Part model, mm, in its own coordinate system. Face numbers are marked on the shaded views. A direction names the side the tool comes from. Coordinates: 2 decimals unless noted, no trailing zeros. Loops run counter-clockwise (first coordinate to the right, second up) from the corner with the lowest first, then second, coordinate; pieces in that order, holes last. Notation, with made-up numbers: (86, 75) - (132, 75) arc R24 ccw to (132, 114) - close; hole circle Ø1 at (15.25, -1). An arc over 180 degrees is marked (long way). Answer as CSV lines item,"result".
from build123d import *

# Parameters (mm, degrees)
SKETCH1_W           = 26
SKETCH1_H           = 41
BOSS_EXTRUDE1_DEPTH = 10
SKETCH2_W           = 26
SKETCH2_H           = 5
BOSS_EXTRUDE2_DEPTH = 25
CUT_EXTRUDE1_REACH  = 73.638
CHAMFER1_SIZE       = 2
SKETCH4_W           = 56
SKETCH4_H           = 8
BOSS_EXTRUDE3_DEPTH = 9
CUT_EXTRUDE2_REACH  = 73.386
SKETCH5_R           = 2.15
SKETCH6_R           = 3.5
CUT_EXTRUDE3_DEPTH  = 5
CHAMFER3_SIZE       = 3
CUT_EXTRUDE5_DEPTH  = 1
CUT_EXTRUDE6_DEPTH  = 4
CUT_EXTRUDE7_REACH  = 73.638
SKETCH12_R          = 1.65
SKETCH14_W          = 12
SKETCH14_H          = 12
CUT_EXTRUDE9_DEPTH  = 7


with BuildPart() as part:
    # Sketch1 → Boss-Extrude1 (new body)
    with BuildSketch(Plane(origin=(0, 0, 0), x_dir=(1, 0, 0), z_dir=(0, 1, 0))):
        with Locations((13, 20.5)):
            Rectangle(SKETCH1_W, SKETCH1_H)
    extrude(amount=BOSS_EXTRUDE1_DEPTH)

    # Sketch2 → Boss-Extrude2 (add)
    with BuildSketch(Plane(origin=(0, 0, -41), x_dir=(-1, 0, 0), z_dir=(0, 0, -1))):
        with Locations((-13, 7.5)):
            Rectangle(SKETCH2_W, SKETCH2_H)
    extrude(amount=BOSS_EXTRUDE2_DEPTH)

    # Sketch3 → Cut-Extrude1 (cut, up to next)
    with BuildSketch(Plane(origin=(0, 10, 0), x_dir=(1, 0, 0), z_dir=(0, 1, 0)), mode=Mode.PRIVATE) as cut_extrude1_sk1:
        with BuildLine():
            Line((0, 56), (0, 66))
            Line((0, 66), (10, 66))
            ThreePointArc((10, 66), (7.071067812, 58.928932188), (0, 56))
        make_face()
    cut_extrude1_tool1 = extrude(cut_extrude1_sk1.sketch, amount=-CUT_EXTRUDE1_REACH, mode=Mode.PRIVATE) & part.part
    add(cut_extrude1_tool1.solids().sort_by_distance((4.244132, 10, -61.755868))[0], mode=Mode.SUBTRACT)

    # Chamfer1
    chamfer1_edges = [part.edges().sort_by_distance(p)[0] for p in [
        (26, 10, -33),
        (18, 10, -66),
        (0, 10, -28),
        (7.071067812, 10, -58.928932188),
        (13, 10, 0),
    ]]
    chamfer(chamfer1_edges, length=CHAMFER1_SIZE)

    # Sketch4 → Boss-Extrude3 (add)
    with BuildSketch(Plane.ZY):
        with Locations((-28, 4)):
            Rectangle(SKETCH4_W, SKETCH4_H)
    extrude(amount=BOSS_EXTRUDE3_DEPTH)

    # Sketch5 → Cut-Extrude2 (cut, up to next)
    with BuildSketch(Plane(origin=(0, 8, 0), x_dir=(1, 0, 0), z_dir=(0, 1, 0)), mode=Mode.PRIVATE) as cut_extrude2_sk1:
        with Locations(Location((-4.5, 51.637478231, 0), (0, 0, 270))):
            Circle(SKETCH5_R)
    cut_extrude2_tool1 = extrude(cut_extrude2_sk1.sketch, amount=-CUT_EXTRUDE2_REACH, mode=Mode.PRIVATE) & part.part
    # Sketch5 → Cut-Extrude2 (cut, up to next)
    with BuildSketch(Plane(origin=(0, 8, 0), x_dir=(1, 0, 0), z_dir=(0, 1, 0)), mode=Mode.PRIVATE) as cut_extrude2_sk2:
        with Locations(Location((-4.5, 4.837478231, 0), (0, 0, 270))):
            Circle(SKETCH5_R)
    cut_extrude2_tool2 = extrude(cut_extrude2_sk2.sketch, amount=-CUT_EXTRUDE2_REACH, mode=Mode.PRIVATE) & part.part
    add(cut_extrude2_tool1.solids().sort_by_distance((-4.5, 8, -51.637478))[0], mode=Mode.SUBTRACT)
    add(cut_extrude2_tool2.solids().sort_by_distance((-4.5, 8, -4.837478))[0], mode=Mode.SUBTRACT)

    # Sketch6 → Cut-Extrude3 (cut)
    with BuildSketch(Plane(origin=(0, 8, 0), x_dir=(1, 0, 0), z_dir=(0, 1, 0))):
        with Locations(Location((-4.5, 51.637478231, 0), (0, 0, 270))):
            Circle(SKETCH6_R)
        with Locations(Location((-4.5, 4.837478231, 0), (0, 0, 270))):
            Circle(SKETCH6_R)
    extrude(amount=-CUT_EXTRUDE3_DEPTH, mode=Mode.SUBTRACT)

    # Chamfer3
    # the kernel refuses this chamfer: 3 mm, written as the material it takes off along each edge
    with BuildSketch(Plane(origin=(-9, 8, -63.715048964), x_dir=(-0.0274958766105862, -0.9996219169112968, 0), z_dir=(0, 0, 1))) as chamfer3_piece_1:
        Polygon((CHAMFER3_SIZE * 0.999621916911, CHAMFER3_SIZE * 0.0274958766106), (-CHAMFER3_SIZE * 0.0274958766106, CHAMFER3_SIZE * 0.999621916911), (0, 0), align=None)
    extrude(amount=71.430097928, mode=Mode.SUBTRACT)

    # Sketch10 → Cut-Extrude5 (cut)
    with BuildSketch(Plane(origin=(0, 10, 0), x_dir=(1, 0, 0), z_dir=(0, 1, 0))):
        Polygon((14.732050808, 39), (13.866025404, 40.5), (12.133974596, 40.5), (11.267949192, 39), (12.133974596, 37.5), (13.866025404, 37.5), align=None)
        Polygon((14.732050808, 43.75), (13.866025404, 45.25), (12.133974596, 45.25), (11.267949192, 43.75), (12.133974596, 42.25), (13.866025404, 42.25), align=None)
        Polygon((17.979646072, 39.875), (18.845671476, 41.375), (17.979646072, 42.875), (16.247595264, 42.875), (15.38156986, 41.375), (16.247595264, 39.875), align=None)
        Polygon((16.247595264, 35.125), (17.979646072, 35.125), (18.845671476, 36.625), (17.979646072, 38.125), (16.247595264, 38.125), (15.38156986, 36.625), align=None)
        Polygon((11.267949192, 34.25), (12.133974596, 32.75), (13.866025404, 32.75), (14.732050808, 34.25), (13.866025404, 35.75), (12.133974596, 35.75), align=None)
        Polygon((8.020353928, 38.125), (7.154328524, 36.625), (8.020353928, 35.125), (9.752404736, 35.125), (10.61843014, 36.625), (9.752404736, 38.125), align=None)
        Polygon((9.752404736, 42.875), (8.020353928, 42.875), (7.154328524, 41.375), (8.020353928, 39.875), (9.752404736, 39.875), (10.61843014, 41.375), align=None)
    extrude(amount=-CUT_EXTRUDE5_DEPTH, mode=Mode.SUBTRACT)

    # Sketch11 → Cut-Extrude6 (cut)
    with BuildSketch(Plane(origin=(0, 10, 0), x_dir=(1, 0, 0), z_dir=(0, 1, 0))):
        Polygon((6.75, 46.08771324), (4, 47.675426481), (1.25, 46.08771324), (1.25, 42.91228676), (4, 41.324573519), (6.75, 42.91228676), align=None)
        Polygon((6.75, 54.08771324), (4, 55.675426481), (1.25, 54.08771324), (1.25, 50.91228676), (4, 49.324573519), (6.75, 50.91228676), align=None)
        Polygon((21.174508901, 58.076331968), (19.521149027, 60.787371337), (16.346640126, 60.711039369), (14.825491099, 57.923668032), (16.478850973, 55.212628663), (19.653359874, 55.288960631), align=None)
    extrude(amount=-CUT_EXTRUDE6_DEPTH, mode=Mode.SUBTRACT)

    # Sketch12 → Cut-Extrude7 (cut, up to next)
    with BuildSketch(Plane(origin=(0, 10, 0), x_dir=(1, 0, 0), z_dir=(0, 1, 0)), mode=Mode.PRIVATE) as cut_extrude7_sk1:
        with Locations(Location((4, 52.5, 0), (0, 0, 270))):
            Circle(SKETCH12_R)
    cut_extrude7_tool1 = extrude(cut_extrude7_sk1.sketch, amount=-CUT_EXTRUDE7_REACH, mode=Mode.PRIVATE) & part.part
    # Sketch12 → Cut-Extrude7 (cut, up to next)
    with BuildSketch(Plane(origin=(0, 10, 0), x_dir=(1, 0, 0), z_dir=(0, 1, 0)), mode=Mode.PRIVATE) as cut_extrude7_sk2:
        with Locations(Location((4, 44.5, 0), (0, 0, 270))):
            Circle(SKETCH12_R)
    cut_extrude7_tool2 = extrude(cut_extrude7_sk2.sketch, amount=-CUT_EXTRUDE7_REACH, mode=Mode.PRIVATE) & part.part
    # Sketch12 → Cut-Extrude7 (cut, up to next)
    with BuildSketch(Plane(origin=(0, 10, 0), x_dir=(1, 0, 0), z_dir=(0, 1, 0)), mode=Mode.PRIVATE) as cut_extrude7_sk3:
        with Locations(Location((18, 58, 0), (0, 0, 270))):
            Circle(SKETCH12_R)
    cut_extrude7_tool3 = extrude(cut_extrude7_sk3.sketch, amount=-CUT_EXTRUDE7_REACH, mode=Mode.PRIVATE) & part.part
    add(cut_extrude7_tool1.solids().sort_by_distance((4, 10, -52.5))[0], mode=Mode.SUBTRACT)
    add(cut_extrude7_tool2.solids().sort_by_distance((4, 10, -44.5))[0], mode=Mode.SUBTRACT)
    add(cut_extrude7_tool3.solids().sort_by_distance((18, 10, -58))[0], mode=Mode.SUBTRACT)

    # Sketch14 → Cut-Extrude9 (cut)
    with BuildSketch(Plane.XZ):
        with Locations((18.75, -23)):
            Rectangle(SKETCH14_W, SKETCH14_H)
    extrude(amount=-CUT_EXTRUDE9_DEPTH, mode=Mode.SUBTRACT)


solid = part.part
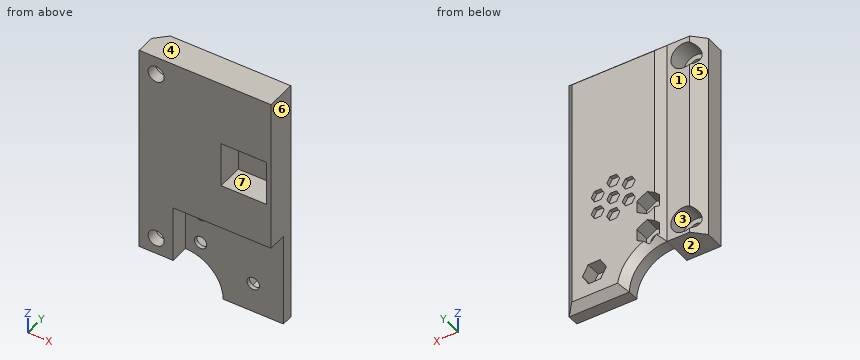
Q1. Saw through at C-C (x = -4.5). Give the cut face in (y, z).
Results:
outline,"(0, -56) - (8, -56) - (8, -55.14) - (3, -55.14) - (3, -53.79) - (0, -53.79) - close; (0, -49.49) - (3, -49.49) - (3, -48.14) - (8, -48.14) - (8, -8.34) - (3, -8.34) - (3, -6.99) - (0, -6.99) - close; (0, -2.69) - (3, -2.69) - (3, -1.34) - (8, -1.34) - (8, 0) - (0, 0) - close"
Q2. Wall check: L1, parallel to Z at x = -4.5, y = 6.25; L2, parallel to X at y = 5.6, z = -58; L3, parallel to Z at x = -6.5, y = 7.25. Give the ranges that are in metal, low to high.
Results:
L1,"z = -56 to -55.14, -48.14 to -8.34, -1.34 to 0"
L2,"x = 6 to 16.35, 19.65 to 26"
L3,"z = -56 to -54.51, -48.77 to -7.71, -1.97 to 0"
Q3. Saw through at B-B (z = -44.5). Give the cut face in (x, y).
Results:
outline,"(-9, 0) - (0, 0) - (0, 5) - (2.35, 5) - (2.35, 6) - (1.25, 6) - (1.25, 9.25) - (0, 8) - (-6, 8) - (-9, 5) - close; (5.65, 5) - (26, 5) - (26, 8) - (24, 10) - (14.3, 10) - (14.3, 9) - (11.7, 9) - (11.7, 10) - (6.75, 10) - (6.75, 6) - (5.65, 6) - close"
Q4. Flat gauge pins, fed straight in: pin 1 (6 mm diameter, centred on x = 21, z = -22.5, fed in from -Y); pin 2 (0.8 mm diameter, centred on x = 8.5, y = 9.5, fed in from -Z); pin 3 (3.5 mm diameter, centred on x = -3, z = -5, fed in from +Y). Where does each tip first touch, or does it go through?
Results:
pin 1,"stops at y = 7"
pin 2,"stops at z = -59.03"
pin 3,"stops at y = 3"
Q5. Saw through at A-A (y = 1.5). Give the cut face in (x, z), then the cut area to 3 significant figures.
Results:
outline,"(-9, -56) - (0, -56) - (0, -41) - (26, -41) - (26, 0) - (-9, 0) - close; hole circle Ø4.3 at (-4.5, -51.64); hole circle Ø4.3 at (-4.5, -4.84); hole (12.75, -29) - (24.75, -29) - (24.75, -17) - (12.75, -17) - close"
area,"1,400 mm^2"
Q6. Which spindle directions (+Z, -Z, +X, -X, +Y, -Y) get a long thin tool onto all of the face, cutting with end or side? Do the marked faces 1, 2 and 3. Say none if no direction does.
Results:
face 1,"+Z, -Z, -X, +Y"
face 2,"-Z, -X, +Y, -Y"
face 3,"+Y"
Q7. Two-plate mould, pull along X, no slides. Class the marked faces 4, 5, 6 and 7: released by +X, released by -X, zero draft, split by the parting line, or undercut.
Results:
face 4,"zero draft"
face 5,"released by -X"
face 6,"released by +X"
face 7,"undercut"
Q8. Saw through at D-D (z = -52.5). Give the cut face in (x, y).
Results:
outline,"(-9, 0) - (-6.47, 0) - (-6.47, 3) - (-7.89, 3) - (-7.89, 6.11) - (-9, 5) - close; (-2.53, 0) - (0, 0) - (0, 5) - (2.35, 5) - (2.35, 6) - (1.25, 6) - (1.25, 9.25) - (0, 8) - (-1.11, 8) - (-1.11, 3) - (-2.53, 3) - close; (5.65, 5) - (26, 5) - (26, 8) - (24, 10) - (6.75, 10) - (6.75, 6) - (5.65, 6) - close"
